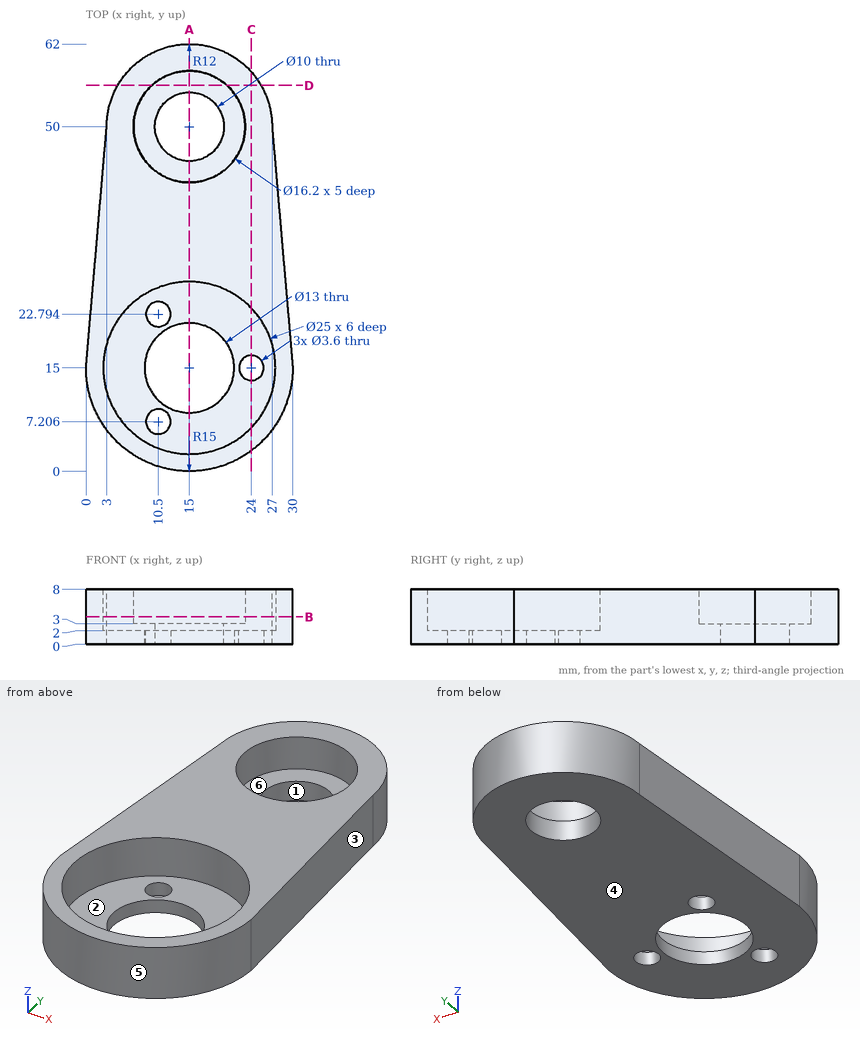
Can you work these out from the drawing? Everything is in mm from the part's minimum corner. A direction names the side the tool comes from. Round coordinates to 2 decimals unless told otherwise and drop trailing zeros. Loops run counter-clockwise (first coordinate to the right, second up) from the corner with the lowest first, then second, coordinate; pieces in that order, holes last. Notation, with made-up numbers: (-26.75, -30) - (-16.75, -30) arc R29 cw to (-16.75, 1) - close; hole circle Ø2 at (0, 10.25). An arc over 180 degrees is marked (long way). Answer in a Markdown table with one row per item. Add a question column.
(1) If we section it at D-D (y = 56): Please give me the cut outline in (x, z).
(2) If we mould it in two halves opening along Y, with no side actions, what happens to the marked faces 1, 2, 3 and 4? For each: pulls with the +Y half, pulls with the -Y half, needs draft (parallel to the pull), parting line crosses it, or undercut.
(3) For the marked faces 5 and 6, which set-ups out of +Z, -Z, +X, -X, +Y, -Y let a thin tool reach every point of the face, with its end or its side?
(4) I'm going to push flat-ended pins straight in: pin 1 (2 mm diameter, centred on x = 10.5, y = 7.21, fed in from -Z); pin 2 (18 mm diameter, centred on x = 16, y = 49, fed in from +Z); pin 3 (1 mm diameter, centred on y = 54.5, z = 5.5, fed in from -X); pin 4 (4 mm diameter, centred on x = 10.5, y = 22.79, fed in from +Z). Where does each tip first touch, or does it pass through?
(5) If we section it at B-B (z = 4): Please give me the cut outline in (x, y).
(6) I need wall thicknesses on line 1 along Y through (x, z) = (15, 1.65); line 2 along Y through (x, z) = (15, 4.95); line 3 along X through (y, z) = (50, 6.75). Which ranges of each line are inside material? Lowest first, please.
(7) If we section it at A-A (x = 15): Please give me the cut outline in (y, z).
(8) If we section it at C-C (x = 24): Please give me the cut outline in (y, z) (1 decimal), plus the area to 3 significant figures.
Model answer:
| question | item | result |
|---|---|---|
| 1 | outline | (4.61, 0) - (25.39, 0) - (25.39, 8) - (20.44, 8) - (20.44, 3) - (9.56, 3) - (9.56, 8) - (4.61, 8) - close |
| 2 | face 1 | undercut |
| 2 | face 2 | undercut |
| 2 | face 3 | pulls with the +Y half |
| 2 | face 4 | needs draft |
| 3 | face 5 | +Z, -Z, -Y |
| 3 | face 6 | +Z |
| 4 | pin 1 | passes through |
| 4 | pin 2 | stops at z = 8 |
| 4 | pin 3 | stops at x = 3.69 |
| 4 | pin 4 | stops at z = 2 |
| 5 | outline | (0, 15) arc R15 ccw to (30, 15) - (27, 50) arc R12 ccw to (3, 50) - close; hole circle Ø25 at (15, 15); hole circle Ø16.2 at (15, 50) |
| 6 | line 1 | y = 0 to 8.5, 21.5 to 45, 55 to 62 |
| 6 | line 2 | y = 0 to 2.5, 27.5 to 41.9, 58.1 to 62 |
| 6 | line 3 | x = 3 to 6.9, 23.1 to 27 |
| 7 | outline | (0, 0) - (8.5, 0) - (8.5, 2) - (2.5, 2) - (2.5, 8) - (0, 8) - close; (21.5, 0) - (45, 0) - (45, 3) - (41.9, 3) - (41.9, 8) - (27.5, 8) - (27.5, 2) - (21.5, 2) - close; (55, 0) - (62, 0) - (62, 8) - (58.1, 8) - (58.1, 3) - (55, 3) - close |
| 8 | outline | (3, 0) - (13.2, 0) - (13.2, 2) - (6.3, 2) - (6.3, 8) - (3, 8) - close; (16.8, 0) - (57.9, 0) - (57.9, 8) - (23.7, 8) - (23.7, 2) - (16.8, 2) - close |
| 8 | area | 328 mm² |
